Here's how the part is built. I have some questions about the finished solid (model axes, mm). Face numbers are marked on the shaded views. A direction names the side the tool comes from. Give positions to 0.01 mm unless a question says otherwise; leave off trailing zeros. Write each loop counter-clockwise with the first axis right and the second up, starting at its lowest first coordinate (ties: lowest second). Pieces come first, ordered by that corner, then holes. Notation, with made-up numbers: (60, -19) - (84, -19) arc R18 cw to (84, -11) - close; hole circle Ø6 at (89, 81). An arc over 180 degrees is marked (long way). Use one line per item in the form item = value. Start each with the question number.
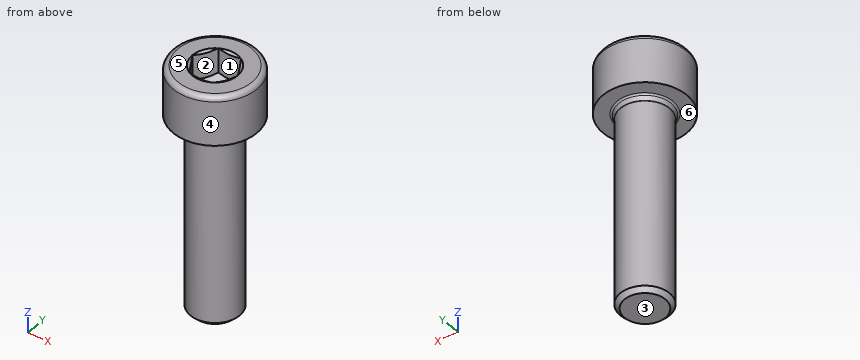
Solid Edge part; units mm, degrees
sketch "Sketch1" plane through (0, 0, 0) normal (0, 0, 1) x (1, 0, 0)
  line L0 (-1.1547, 2) -> (1.1547, 2)
  line L1 (1.1547, 2) -> (2.3094, 0)
  line L2 (2.3094, 0) -> (1.1547, -2)
  line L3 (1.1547, -2) -> (-1.1547, -2)
  line L4 (-1.1547, -2) -> (-2.3094, 0)
  line L5 (-2.3094, 0) -> (-1.1547, 2)
  circle A0 centre (0, 0) radius 4.25
extrude "Protrusion1" add sketch "Sketch1" along normal blind 5
sketch "Sketch2" plane through (0, 0, 0) normal (0, -1, 0) x (1, 0, 0)
  line L0 (0, 1.1667) -> (2.3094, 2.5)
  line L1 (2.3094, 2.5) -> (4.25, 2.5)
  line L2 (4.25, 2.5) -> (4.25, 0)
  line L3 (4.25, 0) -> (2.5, 0)
  line L4 (2.5, 0) -> (2.5, -0.6)
  line L5 (2.5, -0.6) -> (2.5, -0.601) construction
  line L6 (2.5, -0.601) -> (2.5, -0.601) construction
  line L7 (2.5, -0.601) -> (2.5, -20)
  line L8 (0, -20) -> (2.5, -20)
revolve "RevolvedProtrusion_1" add sketch "Sketch2" angle 360 about axis through (0, 0, 2.3333) along (0, 0, -1)
cosmetic_thread "Thread_1" thread depth 19.398
sketch "Sketch3" plane through (0, 0, 0) normal (0, -1, 0) x (1, 0, 0)
  line L0 (0, 6) -> (2.29, 6)
  line L1 (2.29, 6) -> (2.29, 5)
  line L2 (2.29, 5) -> (0, 3.6779)
revolve "RevolvedCutout_1" cut sketch "Sketch3" angle 360 about axis through (0, 0, 7.1999) along (0, 0, 1)
fillet "Round_1" radius 0.5 1 edges at (-4.25, 0, 5)
sketch "Sketch4" plane through (0, 0, 0) normal (0, -1, 0) x (1, 0, 0)
  line L0 (2.5, 0) -> (2.85, 0)
  arc A0 (2.6627, -0.1298) -> (2.85, 0) centre (2.85, -0.2) cw
  line L1 (2.5127, -0.5298) -> (2.6627, -0.1298)
  arc A1 (2.5127, -0.5298) -> (2.5, -0.6) centre (2.7, -0.6) ccw
  line L2 (2.5, 0) -> (2.5, -0.6)
revolve "RevolvedProtrusion_2" add sketch "Sketch4" angle 360 about axis through (0, 0, -1.02) along (0, 0, 1)
chamfer "Chamfer_1" distance 0.433 angle 45 1 edges at (-2.5, 0, -20)
properties material "Steel"
1. For the marked faces 5 and 6, which set-ups out of +Z, -Z, +X, -X, +Y, -Y let a thin tool reach every point of the face, with its end or its side?
2. I want a section at B-B, the plane z = 1.75. List the corners of the cut face in (x, y) for me, then the cut area to 3 significant figures.
3. I want a section at A-A, the plane z = -10.5. List the corners of the cut face in (x, y) for me, then the cut area to 3 significant figures.
4. We'd pull the mould along Y, two halves only. Please class the marked faces 1, 2, 3 and 4: pulls with the +Y half, pulls with the -Y half, needs draft (parallel to the pull), parting line crosses it, or undercut.
5. For P1, Ø5, axis at x = 1.5, z = -9.5, coming from the -Y side; P2, Ø1, axis at x = 1.5, y = -2.5, coming from the -Z side; P3, Ø3, axis at y = 1.5, z = -7.5, coming from the -X side, each with a flat end and sliding along its axis, tell me the tip position at first contact or that it passes through.
6. Please list where these lines run through material, in increasing order: line 1 (Y direction, x = -1, z = -7); line 2 (Z direction, x = -0.25, y = -3.5); line 3 (Y direction, x = -1.5, z = -2.5).
Result sheet:
q1.face_5 = +Z, +X, -X, +Y, -Y
q1.face_6 = -Z
q2.outline = circle Ø8.5 at (0, 0); hole circle Ø2.02 at (0, 0)
q2.area = 53.5 mm2
q3.outline = circle Ø5 at (0, 0)
q3.area = 19.6 mm2
q4.face_1 = undercut
q4.face_2 = undercut
q4.face_3 = needs draft
q4.face_4 = parting line crosses it
q5.P1 = -2.5
q5.P2 = -19.65
q5.P3 = -2.5
q6.line_1 = -2.29 to 2.29
q6.line_2 = 0 to 5
q6.line_3 = -2 to 2
